Autodesk Inventor part; units mm, degrees
ref_plane "YZ Plane" through (0, 0, 0) normal (1, 0, 0) x (0, 1, 0)
ref_plane "XZ Plane" through (0, 0, 0) normal (0, 1, 0) x (-1, 0, 0)
ref_plane "XY Plane" through (0, 0, 0) normal (0, 0, 1) x (1, 0, 0)
sketch "Sketch1" plane through (0, 0, 0) normal (0, 1, 0) x (-1, 0, 0)
  line L0 (-15.494, 12.954) -> (15.494, 12.954)
  line L1 (15.494, 12.954) -> (15.494, -12.954)
  line L2 (15.494, -12.954) -> (-15.494, -12.954)
  line L3 (-15.494, -12.954) -> (-15.494, 12.954)
  line L4 (-15.494, 12.954) -> (15.494, -12.954) construction
  line L5 (15.494, 12.954) -> (-15.494, -12.954) construction
  line L6 (15.494, 12.954) -> (0, 0)
  line L7 (15.494, 12.954) -> (13.462, 12.954)
  line L8 (13.462, 12.954) -> (13.462, 10.922)
  line L9 (13.462, 10.922) -> (15.494, 10.922)
  circle A0 centre (13.462, 10.922) radius 2.032
  line L10 (-15.494, -12.954) -> (-13.462, -12.954)
  line L11 (-13.462, -12.954) -> (-13.462, -10.922)
  line L12 (-13.462, -10.922) -> (-15.494, -10.922)
  line L13 (-15.494, -10.922) -> (-15.494, -12.954)
  line L14 (-15.494, 12.954) -> (-13.462, 12.954)
  line L15 (-13.462, 12.954) -> (-13.462, 10.922)
  line L16 (-13.462, 10.922) -> (-15.494, 10.922)
  line L17 (-15.494, 10.922) -> (-15.494, 12.954)
  line L18 (15.494, -12.954) -> (13.462, -12.954)
  line L19 (13.462, -12.954) -> (13.462, -10.922)
  line L20 (13.462, -10.922) -> (15.494, -10.922)
  line L21 (15.494, -10.922) -> (15.494, -12.954)
  circle A1 centre (13.462, -10.922) radius 2.032
  circle A2 centre (-13.462, 10.922) radius 2.032
  circle A3 centre (-13.462, -10.922) radius 2.032
  circle A4 centre (-13.462, 10.922) radius 1.5367
  circle A5 centre (13.462, 10.922) radius 1.5367
  circle A6 centre (13.462, -10.922) radius 1.5367
  circle A7 centre (-13.462, -10.922) radius 1.5367
  dimension "d0" = 30.988
  dimension "d1" = 25.908
  dimension "d2" = 2.032
  dimension "d3" = 2.032
  dimension "d4" = 2.032
  dimension "d5" = 2.032
  dimension "d6" = 3.0734
extrude "Extrusion1" add sketch "Sketch1" along normal blind 2.794 contours A2 L16 A4 L15 | L0 A0 L1 A1 L2 A3 L3 A2 | L15 A4 L16 A2 | A0 L6 A5 L8 | L8 A5 L6 A0 | A3 L11 A7 L12 | L12 A7 L11 A3 | A0 L9 A5 L6 | L6 A5 L9 A0 | A1 L20 A6 L19 | L19 A6 L20 A1
sketch "Sketch2" plane through (0, 2.794, 0) normal (0, 1, 0) x (1, 0, 0)
  circle A0 centre (-13.462, 10.922) radius 1.5367
  circle A1 centre (-13.462, 10.922) radius 1.5367
  circle A2 centre (13.462, -10.922) radius 1.5367
  circle A3 centre (13.462, -10.922) radius 1.5367
  point P0 (0, 0)
extrude "Extrusion2" add sketch "Sketch2" against normal blind 2.794
sketch "Sketch3" plane through (0, 2.794, 0) normal (0, 1, 0) x (1, 0, 0)
  circle A0 centre (0, 0) radius 11.7856
  dimension "d11" = 23.5712
extrude "Extrusion3" add sketch "Sketch3" along normal blind 3.429
sketch "Sketch4" plane through (0, 0, 0) normal (0, -1, 0) x (1, 0, 0)
  circle A0 centre (0, 0) radius 10.8712
  dimension "d14" = 21.7424
extrude "Extrusion4" add sketch "Sketch4" along normal blind 11.3792
sketch "Sketch5" plane through (0, -11.3792, 0) normal (0, -1, 0) x (1, 0, 0)
  circle A0 centre (0, 0) radius 9.5631
  dimension "d17" = 19.1262
extrude "Extrusion5" add sketch "Sketch5" along normal blind 14.2494
sketch "Sketch6" plane through (0, 6.223, 0) normal (0, 1, 0) x (1, 0, 0)
  line L0 (5.715, -5.715) -> (-5.715, -5.715)
  line L1 (-5.715, -5.715) -> (-5.715, 5.715)
  line L2 (-5.715, 5.715) -> (5.715, 5.715)
  line L3 (5.715, 5.715) -> (5.715, -5.715)
  line L4 (5.715, -5.715) -> (-5.715, 5.715) construction
  line L5 (-5.715, -5.715) -> (5.715, 5.715) construction
  point P0 (0, 0)
  dimension "d20" = 11.43
  dimension "d21" = 11.43
extrude "Extrusion6" cut sketch "Sketch6" against normal blind 0.0254
sketch "Sketch7" plane through (0, 6.1976, 0) normal (0, 1, 0) x (1, 0, 0)
  line L0 (4.8156, -4.768) -> (-4.8156, -4.768)
  line L1 (-4.8156, -4.768) -> (-4.8156, 4.768)
  line L2 (-4.8156, 4.768) -> (4.8156, 4.768)
  line L3 (4.8156, 4.768) -> (4.8156, -4.768)
  line L4 (4.8156, -4.768) -> (-4.8156, 4.768) construction
  line L5 (-4.8156, -4.768) -> (4.8156, 4.768) construction
  line L6 (4.8156, -4.768) -> (4.8156, 0)
  line L7 (4.8156, -2.384) -> (2.4316, -4.768)
  line L8 (4.8156, -2.384) -> (8.1872, -2.384) construction
  line L9 (4.8156, 0) -> (4.8156, 4.768)
  line L10 (4.8156, 2.384) -> (2.4316, 4.768)
  line L11 (4.8156, 2.384) -> (8.1872, 2.384) construction
  point P0 (0, 0)
  dimension "d24" = 135
  dimension "d25" = 135
extrude "Extrusion7" cut sketch "Sketch7" against normal blind 8.89 contours L0 L1 L2 L10 L3 L7
sketch "Sketch8" plane through (0, -2.6924, 0) normal (0, 1, 0) x (1, 0, 0)
  line L0 (-2.2203, -3.589) -> (2.2203, -3.589)
  line L1 (2.2203, -3.589) -> (2.2203, 3.589)
  line L2 (2.2203, 3.589) -> (-2.2203, 3.589)
  line L3 (-2.2203, 3.589) -> (-2.2203, -3.589)
  line L4 (-2.2203, -3.589) -> (2.2203, 3.589) construction
  line L5 (2.2203, -3.589) -> (-2.2203, 3.589) construction
  point P0 (0, 0)
extrude "Extrusion8" add sketch "Sketch8" along normal blind 8.89
chamfer "Chamfer1" distance 0.508 angle 45 2 edges at (-11.9253, 2.794, 10.922) (14.9987, 2.794, -10.922)
properties part number "USB Type B Socket"
Verification items for the finished model (mm, model axes). A direction names the side the tool comes from. Give positions to 0.01 mm unless a question says otherwise; leave off trailing zeros. Write each loop counter-clockwise with the first axis right and the second up, starting at its lowest first coordinate (ties: lowest second). Pieces come first, ordered by that corner, then holes.
(1) Access from +Z, -Z, +X, -X, +Y, -Y to the whole of each face (thin tool, end or side, straight path). Record for faces 1 (the face through (11, 2.794, 6)), 2 (the face through (11, 0, 3)), 3 (the face through (-14.883, 1.371, 12.375)).
(2) Cross-section at B-B (z = 0). Enter the section's corners in (x, y) (3 decimals), plus the area to 3 significant figures.
(3) Gauge pin test, flat ends, axial feed: pin 1 (10 mm diameter, centred on x = -9, y = -22, fed in from -Z); pin 2 (3 mm diameter, centred on x = 1, z = 0.5, fed in from +Y); pin 3 (4 mm diameter, centred on x = -13.462, z = 10.922, fed in from -Y). Record the tip position at first contact, or that the pin passes through.
(4) Cross-section at A-A (y = 1.5). Enter the section's corners in (x, z).
(5) Cross-section at D-D (y = -18.5). Enter the section's corners in (x, z), plus the area to 3 significant figures.
(6) Material ranges on line 1 (X direction, y = -0.5, z = -2.25); line 2 (Y direction, x = 11, z = 1); line 3 (X direction, y = -14.5, z = 0.25), recorded low to high.
(7) Cross-section at C-C (x = 0). Enter the section's corners in (y, z) (3 decimals).
(8) Mould release check, pull along X, two halves, no side actions. Record for faces 4 (the face through (-13.26, 1.13, 9.4)), 5 (the face through (11.24, 4.48, 3.54)): +X half, -X half, draft (parallel to the pull), parting line (faces both ways), or undercut.
Worked out:
1. face 1: +Y
1. face 2: -Y
1. face 3: +Z, -X, +Y, -Y
2. outline: (-15.494, 0) - (-10.871, 0) - (-10.871, -11.379) - (-9.563, -11.379) - (-9.563, -25.629) - (9.563, -25.629) - (9.563, -11.379) - (10.871, -11.379) - (10.871, 0) - (15.494, 0) - (15.494, 2.794) - (11.786, 2.794) - (11.786, 6.223) - (5.715, 6.223) - (5.715, 6.198) - (4.816, 6.198) - (4.816, -2.692) - (2.22, -2.692) - (2.22, 6.198) - (-2.22, 6.198) - (-2.22, -2.692) - (-4.816, -2.692) - (-4.816, 6.198) - (-5.715, 6.198) - (-5.715, 6.223) - (-11.786, 6.223) - (-11.786, 2.794) - (-15.494, 2.794) - close
2. area: 641 mm2
3. pin 1: stops at z = -8.69
3. pin 2: stops at y = 6.2
3. pin 3: stops at y = 0
4. outline: (-15.49, -10.92) arc R2.03 ccw to (-13.46, -12.95) - (13.46, -12.95) arc R2.03 ccw to (15.49, -10.92) - (15.49, 10.92) arc R2.03 ccw to (13.46, 12.95) - (-13.46, 12.95) arc R2.03 ccw to (-15.49, 10.92) - close; (-2.22, -3.59) - (2.22, -3.59) - (2.22, 3.59) - (-2.22, 3.59) - close; hole circle Ø3.07 at (-13.46, 10.92); hole (-4.82, -4.77) - (2.43, -4.77) - (4.82, -2.38) - (4.82, 2.38) - (2.43, 4.77) - (-4.82, 4.77) - close; hole circle Ø3.07 at (13.46, -10.92)
5. outline: circle Ø19.13 at (0, 0)
5. area: 287 mm2
6. line 1: x = -10.64 to -4.82, -2.22 to 2.22, 4.82 to 10.64
6. line 2: y = 0 to 6.22
6. line 3: x = -9.56 to 9.56
7. outline: (-25.629, -9.563) - (-11.379, -9.563) - (-11.379, -10.871) - (0, -10.871) - (0, -12.954) - (2.794, -12.954) - (2.794, -11.786) - (6.223, -11.786) - (6.223, -5.715) - (6.198, -5.715) - (6.198, -4.768) - (-2.692, -4.768) - (-2.692, -3.589) - (6.198, -3.589) - (6.198, 3.589) - (-2.692, 3.589) - (-2.692, 4.768) - (6.198, 4.768) - (6.198, 5.715) - (6.223, 5.715) - (6.223, 11.786) - (2.794, 11.786) - (2.794, 12.954) - (0, 12.954) - (0, 10.871) - (-11.379, 10.871) - (-11.379, 9.563) - (-25.629, 9.563) - close
8. face 4: undercut
8. face 5: parting line
